Source: CAD feature listing. Evaluate the final solid. Frame: model axes, mm. Face numbers are marked on the shaded views. A direction names the side the tool comes from. Coordinates: 2 decimals unless noted, no trailing zeros. Order: outer loops, then holes, each group sorted by start corner. A loop starts at its lowest first (then second) coordinate and runs counter-clockwise, first axis right, second up. Notation, with made-up numbers: (68, -5.5) -> (124, -5.5) arc R21 ccw to (124, 22.5) -> close; hole circle Ø3 at (14, 35.5). An arc over 180 degrees is marked (long way). Put each result on its own line as item: value.
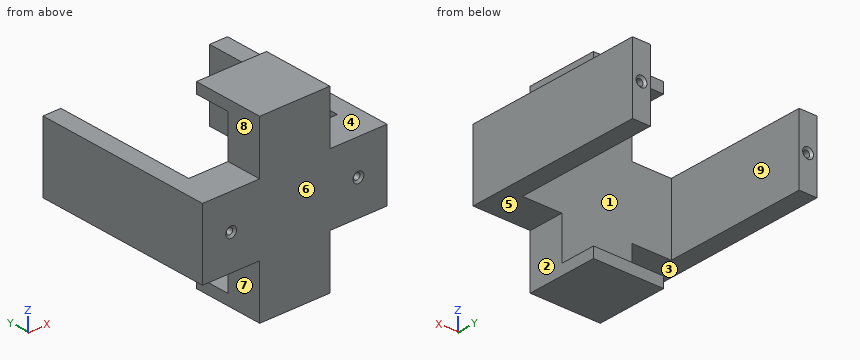
from build123d import *

# Parameters (mm, degrees)
RESSALTO_EXTRUS_O1_DEPTH                             = 10
ESBO_O2_W                                            = 5
ESBO_O2_H                                            = 19.6
RESSALTO_EXTRUS_O2_DEPTH                             = 50.4
RESSALTO_EXTRUS_O3_DEPTH                             = 10
RESSALTO_EXTRUS_O3_DEPTH_BACK                        = 10
ESBO_O3_W                                            = 19.6
ESBO_O3_H                                            = 3
ESCAREADO_PARA_PARAFUSO_DE_M_QUINA_COM_C_D           = 1.778
ESCAREADO_PARA_PARAFUSO_DE_M_QUINA_COM_C_DEPTH       = 5
ESCAREADO_PARA_PARAFUSO_DE_M_QUINA_COM_C_CSINK_D     = 3.0226
ESCAREADO_PARA_PARAFUSO_DE_M_QUINA_COM_C_CSINK_ANGLE = 100
ESCAREADO_PARA_PARAFUSO_DE_M_QUINA_COM_C_TIP         = 0.53416509
ESCAREADO_PARA_PARAFUSO_DE_M_QUINA_C_2_D             = 1.778
ESCAREADO_PARA_PARAFUSO_DE_M_QUINA_C_2_DEPTH         = 5
ESCAREADO_PARA_PARAFUSO_DE_M_QUINA_C_2_CSINK_D       = 3.0226
ESCAREADO_PARA_PARAFUSO_DE_M_QUINA_C_2_CSINK_ANGLE   = 100
ESCAREADO_PARA_PARAFUSO_DE_M_QUINA_C_2_TIP           = 0.53416509


with BuildPart() as part:
    # Esboço1 → Ressalto-extrusão1 (new body)
    with BuildSketch(Plane(origin=(0, 0, 0), x_dir=(1, 0, 0), z_dir=(0, 1, 0))):
        Polygon((-9.8, 21.8), (-9.8, 9.8), (-20.8, 9.8), (-20.8, -9.8), (-9.8, -9.8), (-9.8, -21.8), (9.8, -21.8), (9.8, -9.8), (20.8, -9.8), (20.8, 9.8), (9.8, 9.8), (9.8, 21.8), align=None)
    extrude(amount=RESSALTO_EXTRUS_O1_DEPTH)

    # Esboço2 → Ressalto-extrusão2 (add)
    with BuildSketch(Plane(origin=(0, 0, 0), x_dir=(1, 0, 0), z_dir=(0, 1, 0))):
        with Locations((23.3, 0)):
            Rectangle(ESBO_O2_W, ESBO_O2_H)
        with Locations((-23.3, 0)):
            Rectangle(ESBO_O2_W, ESBO_O2_H)
    extrude(amount=RESSALTO_EXTRUS_O2_DEPTH)

    # Esboço3 → Ressalto-extrusão3 (add, two sides: drawn at the far end of the back side and taken through both)
    with BuildSketch(Plane(origin=(0, 10, 0), x_dir=(1, 0, 0), z_dir=(0, 1, 0)).offset(-RESSALTO_EXTRUS_O3_DEPTH_BACK)):
        with Locations((0, 23.3)):
            Rectangle(ESBO_O3_W, ESBO_O3_H)
        with Locations((0, -23.3)):
            Rectangle(ESBO_O3_W, ESBO_O3_H)
    extrude(amount=RESSALTO_EXTRUS_O3_DEPTH + RESSALTO_EXTRUS_O3_DEPTH_BACK)

    # Escareado para parafuso de m_quina com c
    with Locations(Plane(origin=(0, 50.4, 0), x_dir=(1, 0, 0), z_dir=(0, 1, 0))):
        with Locations((-23.3, 0), (23.3, 0)):
            CounterSinkHole(ESCAREADO_PARA_PARAFUSO_DE_M_QUINA_COM_C_D / 2, ESCAREADO_PARA_PARAFUSO_DE_M_QUINA_COM_C_CSINK_D / 2, depth=ESCAREADO_PARA_PARAFUSO_DE_M_QUINA_COM_C_DEPTH, counter_sink_angle=ESCAREADO_PARA_PARAFUSO_DE_M_QUINA_COM_C_CSINK_ANGLE)
            with Locations((0, 0, -(ESCAREADO_PARA_PARAFUSO_DE_M_QUINA_COM_C_DEPTH + ESCAREADO_PARA_PARAFUSO_DE_M_QUINA_COM_C_TIP / 2))):  # 118° drill point
                Cone(0, ESCAREADO_PARA_PARAFUSO_DE_M_QUINA_COM_C_D / 2, ESCAREADO_PARA_PARAFUSO_DE_M_QUINA_COM_C_TIP, mode=Mode.SUBTRACT)

    # Escareado para parafuso de m_quina c 2
    with Locations(Plane(origin=(0, 0, 0), x_dir=(-1, 0, 0), z_dir=(0, -1, 0))):
        with Locations((-17.8, 0), (17.8, 0)):
            CounterSinkHole(ESCAREADO_PARA_PARAFUSO_DE_M_QUINA_C_2_D / 2, ESCAREADO_PARA_PARAFUSO_DE_M_QUINA_C_2_CSINK_D / 2, depth=ESCAREADO_PARA_PARAFUSO_DE_M_QUINA_C_2_DEPTH, counter_sink_angle=ESCAREADO_PARA_PARAFUSO_DE_M_QUINA_C_2_CSINK_ANGLE)
            with Locations((0, 0, -(ESCAREADO_PARA_PARAFUSO_DE_M_QUINA_C_2_DEPTH + ESCAREADO_PARA_PARAFUSO_DE_M_QUINA_C_2_TIP / 2))):  # 118° drill point
                Cone(0, ESCAREADO_PARA_PARAFUSO_DE_M_QUINA_C_2_D / 2, ESCAREADO_PARA_PARAFUSO_DE_M_QUINA_C_2_TIP, mode=Mode.SUBTRACT)


solid = part.part
1. Cut plane B-B on z = 8. Output: boundary loops of the cut face in (x, y).
Numbers:
outline: (-25.8, 0) -> (25.8, 0) -> (25.8, 50.4) -> (20.8, 50.4) -> (20.8, 10) -> (-20.8, 10) -> (-20.8, 50.4) -> (-25.8, 50.4) -> close
2. Cut plane A-A on y = 18.5. Output: boundary loops of the cut face in (x, z).
Numbers:
outline: (-25.8, -9.8) -> (-20.8, -9.8) -> (-20.8, 9.8) -> (-25.8, 9.8) -> close; (-9.8, -24.8) -> (9.8, -24.8) -> (9.8, -21.8) -> (-9.8, -21.8) -> close; (-9.8, 21.8) -> (9.8, 21.8) -> (9.8, 24.8) -> (-9.8, 24.8) -> close; (20.8, -9.8) -> (25.8, -9.8) -> (25.8, 9.8) -> (20.8, 9.8) -> close
3. First-contact query: pin 1 (8 mm diameter, centred on x = -16, z = 13, fed in from +Y); pin 2 (17.5 mm diameter, centred on x = -18, y = 33, fed in from -Z); pin 3 (2.5 mm diameter, centred on x = -4.5, z = 23, fed in from +Y). Flat tips, straight axial feed; report the tip coordinate or a pass-through.
Numbers:
pin 1: stops at y = 10
pin 2: stops at z = -9.8
pin 3: stops at y = 20
4. Ray query, line 1 along X through (y, z) = (28.5, -7.5); line 2 along Z through (x, y) = (-17.8, 2.4); line 3 along Z through (x, y) = (-21.5, 18). Return the intervals inside material, ascending.
Numbers:
line 1: x = -25.8 to -20.8, 20.8 to 25.8
line 2: z = -9.8 to -0.89, 0.89 to 9.8
line 3: z = -9.8 to 9.8
5. Cut plane C-C on x = -7. Output: boundary loops of the cut face in (y, z), plus the area to 3 significant figures.
Numbers:
outline: (0, -24.8) -> (20, -24.8) -> (20, -21.8) -> (10, -21.8) -> (10, 21.8) -> (20, 21.8) -> (20, 24.8) -> (0, 24.8) -> close
area: 556 mm2
6. Cut plane D-D on z = -13. Output: boundary loops of the cut face in (x, y), plus the area to 3 significant figures.
Numbers:
outline: (-9.8, 0) -> (9.8, 0) -> (9.8, 10) -> (-9.8, 10) -> close
area: 196 mm2
7. Pull-direction query (Z, two-part tool) for the marked faces 1, 2, 3 and 4; classes: pulls with the +Z half, pulls with the -Z half, needs draft (parallel to the pull), parting line crosses it, or undercut.
Numbers:
face 1: undercut
face 2: needs draft
face 3: pulls with the -Z half
face 4: pulls with the +Z half
8. Set-up query: the marked faces 5, 6, 7, 8 and 9. Return all of +Z, -Z, +X, -X, +Y, -Y with unobstructed straight access to the full face (end or side cutting, diameter ignored); none if empty.
Numbers:
face 5: -Z, +X, +Y, -Y
face 6: +Z, -Z, +X, -X, -Y
face 7: -Z, -X, +Y, -Y
face 8: +Z, -X, +Y, -Y
face 9: +Z, -Z, +Y
